from build123d import *

# Parameters (mm, degrees)
ESQUISSE1_W             = 1.5
ESQUISSE1_H             = 22
ENL_V_MAT_EXTRU_1_DEPTH = 1.5
ENL_V_START             = -1.5
ENL_V_MAT_EXTRU_2_DEPTH = 1.5
CHANFREIN1_SIZE         = 0.1
CHANFREIN2_SIZE         = 0.1


with BuildPart() as part:
    # Esquisse1 → Révolution1 (revolve)
    with BuildSketch(Plane.XY.offset(10.4), mode=Mode.PRIVATE) as r_volution1_sk:
        with Locations((22.507807929, -2.312735583)):
            Rectangle(ESQUISSE1_W, ESQUISSE1_H)
    revolve(r_volution1_sk.sketch.rotate(Axis((21.757807929, 8.687264417, 10.4), (0, -1, 0)), 270), axis=Axis((21.757807929, 8.687264417, 10.4), (0, -1, 0)))

    # Esquisse2 → Enlèv. mat.-Extru.1 (cut)
    with BuildSketch(Plane(origin=(0, 8.687264417, 0), x_dir=(-1, 0, 0), z_dir=(0, 1, 0))):
        with BuildLine():
            Line((-23.026665683, 11.2), (-20.488950175, 11.2))
            ThreePointArc((-20.488950175, 11.2), (-21.757807929, 11.9), (-23.026665683, 11.2))
        make_face()
    extrude(amount=-ENL_V_MAT_EXTRU_1_DEPTH, mode=Mode.SUBTRACT)

    # Esquisse3 → Enlèv. mat.-Extru.2 (cut)
    with BuildSketch(Plane.XZ.offset(13.312735583).offset(ENL_V_START)):
        with BuildLine():
            Line((20.488950175, 11.2), (23.026665683, 11.2))
            ThreePointArc((23.026665683, 11.2), (21.757807929, 11.9), (20.488950175, 11.2))
        make_face()
    extrude(amount=ENL_V_MAT_EXTRU_2_DEPTH, mode=Mode.SUBTRACT)

    # Chanfrein1
    chanfrein1_edges = [part.edges().sort_by_distance(p)[0] for p in [
        (20.444415375, 8.687264417, 9.675431163),
    ]]
    chamfer(chanfrein1_edges, length=CHANFREIN1_SIZE)

    # Chanfrein2
    chanfrein2_edges = [part.edges().sort_by_distance(p)[0] for p in [
        (23.071200482, -13.312735583, 9.675431163),
    ]]
    chamfer(chanfrein2_edges, length=CHANFREIN2_SIZE)


solid = part.part
Verification items for the finished model (mm, model axes). A direction names the side the tool comes from. Coordinates: 2 decimals unless noted, no trailing zeros. Order: outer loops, then holes, each group sorted by start corner. A loop starts at its lowest first (then second) coordinate and runs counter-clockwise, first axis right, second up. Notation, with made-up numbers: M 82,-10 L 125,-10 A25 cw 125,26 Z; hole C -31,87 d3. An arc over 180 degrees is marked long. One line per item, written item: value. Start each with the question number.
Item 1: Sectioned sample at A-A (z = 11.55). Enter the section's corners in (x, y), then the cut area to 3 significant figures.
Item 2: Scan lines: probe 1 along Y at (x, z) = (22.45, 11.55); probe 2 along Z at (x, y) = (23.05, 6.5); probe 3 along X at (y, z) = (2.5, 10.5). Record each from-to range of solid material in increasing order.
Item 3: Sectioned sample at B-B (y = -8.25). Enter the section's corners in (x, z), then the cut area to 3 significant figures.
Item 4: Access from +Z, -Z, +X, -X, +Y, -Y to the whole of each face (thin tool, end or side, straight path). Record for faces 1 (the flat face through (22, 8.687, 10)), 2 (the flat face through (22, -13, 11.2)), 3 (the flat face through (22, 8, 11.2)).
Item 5: Gauge pin test, flat ends, axial feed: pin 1 (1 mm diameter, centred on y = -0.5, z = 11, fed in from +X); pin 2 (1 mm diameter, centred on y = 3, z = 9.5, fed in from +X); pin 3 (0.8 mm diameter, centred on x = 22, y = 8, fed in from +Z). Record the tip position at first contact, or that the pin passes through.
Conclusion:
1. outline: M 20.79,-11.81 L 22.72,-11.81 L 22.72,7.19 L 20.79,7.19 Z
1. area: 36.6 mm^2
2. probe 1: y = -11.81 to 7.19
2. probe 2: z = 9.64 to 11.16
2. probe 3: x = 20.26 to 23.25
3. outline: C 21.76,10.4 d3
3. area: 7.07 mm^2
4. face 1: +Z, -Z, +X, -X, +Y
4. face 2: +Z, +X, -X, -Y
4. face 3: +Z, +X, -X, +Y
5. pin 1: stops at x = 23.25
5. pin 2: stops at x = 23.2
5. pin 3: stops at z = 11.2
